from build123d import *

# Parameters (mm, degrees)
SKETCH1_R           = 14.2748
BOSS_EXTRUDE1_DEPTH = 6.35


with BuildPart() as part:
    # Sketch1 → Boss-Extrude1 (new body)
    with BuildSketch(Plane(origin=(0, 0, 0), x_dir=(1, 0, 0), z_dir=(0, 1, 0))):
        with BuildLine():
            Line((0, 0), (0, 406.4))
            Line((0, 406.4), (50.8, 406.4))
            Line((50.8, 406.4), (50.8, 0))
            ThreePointArc((50.8, 0), (43.360512242, -17.960512242), (25.4, -25.4))
            ThreePointArc((25.4, -25.4), (7.439487758, -17.960512242), (0, 0))
        make_face()
        with Locations((25.4, 0)):
            Circle(SKETCH1_R, mode=Mode.SUBTRACT)
        with Locations((25.4, 381)):
            Circle(SKETCH1_R, mode=Mode.SUBTRACT)
    extrude(amount=BOSS_EXTRUDE1_DEPTH)


solid = part.part
Geometry check sheet. Reference: the model listing, model coordinates, mm. Give positions to 0.01 mm unless a question says otherwise; leave off trailing zeros. Write each loop counter-clockwise with the first axis right and the second up, starting at its lowest first coordinate (ties: lowest second). Pieces come first, ordered by that corner, then holes.
1) Cross-section at B-B (y = 1). Record the boundary of the cut face in (x, z), plus the area to 3 significant figures.
Values follow:
outline: (0, -406.4) - (50.8, -406.4) - (50.8, 0) arc R25.4 ccw to (0, 0) - close; hole circle Ø28.55 at (25.4, -381); hole circle Ø28.55 at (25.4, 0)
area: 20,400 mm2
2) Cross-section at C-C (x = 32). Record the boundary of the cut face in (y, z).
Values follow:
outline: (0, -406.4) - (6.35, -406.4) - (6.35, -393.66) - (0, -393.66) - close; (0, -368.34) - (6.35, -368.34) - (6.35, -12.66) - (0, -12.66) - close; (0, 12.66) - (6.35, 12.66) - (6.35, 24.53) - (0, 24.53) - close
3) Cross-section at A-A (z = -381). Record the boundary of the cut face in (x, y).
Values follow:
outline: (0, 0) - (11.13, 0) - (11.13, 6.35) - (0, 6.35) - close; (39.67, 0) - (50.8, 0) - (50.8, 6.35) - (39.67, 6.35) - close
4) Thickness scan on line 1 (Z direction, x = 25.4, y = 4.75); line 2 (X direction, y = 5.25, z = -381); line 3 (Z direction, x = 28, y = 2.75). Record the ranges inside material, lowest first.
Values follow:
line 1: z = -406.4 to -395.27, -366.73 to -14.27, 14.27 to 25.4
line 2: x = 0 to 11.13, 39.67 to 50.8
line 3: z = -406.4 to -395.04, -366.96 to -14.04, 14.04 to 25.27
5) Release check for a two-part mould opening along Z. For faces 1 (the face through (26, 0, -194)), 2 (the face through (31.987, 3.131, -368.336)) record: released by +Z, released by -Z, zero draft, split by the parting line, or undercut.
Values follow:
face 1: zero draft
face 2: undercut
